Check sheet for the modelled part. Datum: model origin and axes. Units: mm. Face numbers are marked on the shaded views. Coordinates: 2 decimals unless noted, no trailing zeros. Order: outer loops, then holes, each group sorted by start corner. A loop starts at its lowest first (then second) coordinate and runs counter-clockwise, first axis right, second up.
1. Thickness scan on line 1 (Z direction, x = 0, y = 40); line 2 (Z direction, x = -13.5, y = 60.5); line 3 (X direction, y = 46.5, z = 4). Record the ranges inside material, lowest first.
2. Cross-section at C-C (y = 120). Enter the section's corners in (x, z).
3. Gauge pin test, flat ends, axial feed: pin 1 Ø2 at (y, z) = (100.5, 7) entering from +X; pin 2 Ø1 at (y, z) = (79, -4.5) entering from -X; pin 3 Ø1 at (x, y) = (-8, 102.5) entering from -Z. Record the tip position at first contact, or that the pin passes through.
4. Draft check along X on the marked faces 1 and 2. Enter one of: released by +X, released by -X, zero draft, split by the parting line, or undercut.
```python
from build123d import *

# Parameters (mm, degrees)
F0_R     = 25
F0_R_2   = 15
F1_DEPTH = 130
F2_R     = 4.99999


# Not quite as in the source:
# - a fillet or chamfer is up to 0.001 mm smaller than in the source, because OpenCascade refuses the exact size


with BuildPart() as f1:
    # F0 (on Front) → F1 (new body)
    with BuildSketch(Plane.XZ):
        Circle(F0_R)
        Circle(F0_R_2, mode=Mode.SUBTRACT)
    extrude(amount=-F1_DEPTH)

    # F2 (radius 5 in the source; OpenCascade refuses exactly that, so slightly less here)
    f2_edges = [f1.edges().sort_by_distance(p)[0] for p in [
        (-15, 0, 0),
        (-25, 0, 0),
        (25, 65, 0),
        (-25, 130, 0),
        (-15, 130, 0),
    ]]
    fillet(f2_edges, radius=F2_R)


solid = f1.part
```
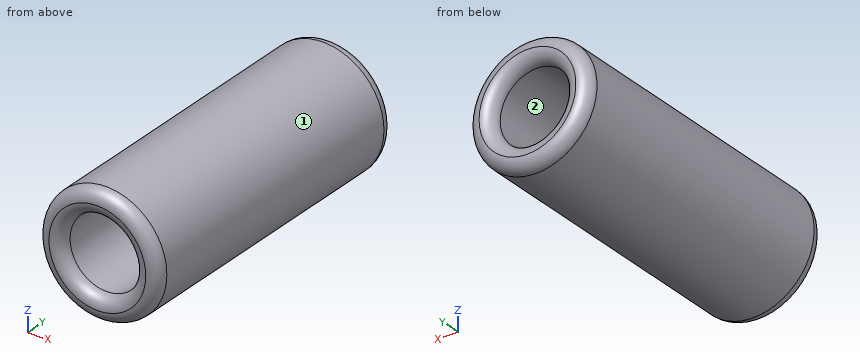
Data:
1. line 1: z = -25 to -15, 15 to 25
1. line 2: z = -21.04 to -6.54, 6.54 to 21.04
1. line 3: x = -24.68 to -14.46, 14.46 to 24.68
2. outline: circle Ø50 at (0, 0); hole circle Ø30 at (0, 0)
3. pin 1: stops at x = 24.27
3. pin 2: stops at x = -24.68
3. pin 3: stops at z = -23.85
4. face 1: split by the parting line
4. face 2: undercut
